from build123d import *

# Parameters (mm, degrees)
F0_R     = 60
F1_DEPTH = 30


with BuildPart() as f1:
    # F0 (on Front) → F1 (new body)
    with BuildSketch(Plane.XZ):
        Polygon((-55, 79.594996), (-125, 79.594996), (-125, 29.594996), (-125, -30.405004), (-125, -80.405004), (-55, -80.405004), (45, -80.405004), (115, -80.405004), (115, -30.405004), (115, 29.594996), (115, 79.594996), (45, 79.594996), align=None)
        with BuildLine():
            ThreePointArc((-110, 55.243649), (-107.071068, 62.314716), (-100, 65.243649))
            Line((-100, 65.243649), (-90, 65.243649))
            ThreePointArc((-90, 65.243649), (-82.928932, 62.314716), (-80, 55.243649))
            Line((-80, 55.243649), (-80, -54.756351))
            ThreePointArc((-80, -54.756351), (-82.928932, -61.827419), (-90, -64.756351))
            Line((-90, -64.756351), (-100, -64.756351))
            ThreePointArc((-100, -64.756351), (-107.071068, -61.827419), (-110, -54.756351))
            Line((-110, -54.756351), (-110, 55.243649))
        make_face(mode=Mode.SUBTRACT)
        Circle(F0_R, mode=Mode.SUBTRACT)
        with BuildLine():
            ThreePointArc((80, 55.243649), (82.928932, 62.314716), (90, 65.243649))
            Line((90, 65.243649), (100, 65.243649))
            ThreePointArc((100, 65.243649), (107.071068, 62.314716), (110, 55.243649))
            Line((110, 55.243649), (110, -54.756351))
            ThreePointArc((110, -54.756351), (107.071068, -61.827419), (100, -64.756351))
            Line((100, -64.756351), (90, -64.756351))
            ThreePointArc((90, -64.756351), (82.928932, -61.827419), (80, -54.756351))
            Line((80, -54.756351), (80, 55.243649))
        make_face(mode=Mode.SUBTRACT)
        with BuildLine():
            Line((-125, -30.405004), (-125, 29.594996))
            ThreePointArc((-125, 29.594996), (-148.860331, -0.405004), (-125, -30.405004))
        make_face()
        with BuildLine():
            ThreePointArc((45, 79.594996), (-5, 105.335071), (-55, 79.594996))
            Line((-55, 79.594996), (45, 79.594996))
        make_face()
        with BuildLine():
            Line((45, -80.405004), (-55, -80.405004))
            ThreePointArc((-55, -80.405004), (-5, -106.628586), (45, -80.405004))
        make_face()
        with BuildLine():
            ThreePointArc((115, -30.405004), (136.54259, -0.405004), (115, 29.594996))
            Line((115, 29.594996), (115, -30.405004))
        make_face()
    extrude(amount=F1_DEPTH)


solid = f1.part
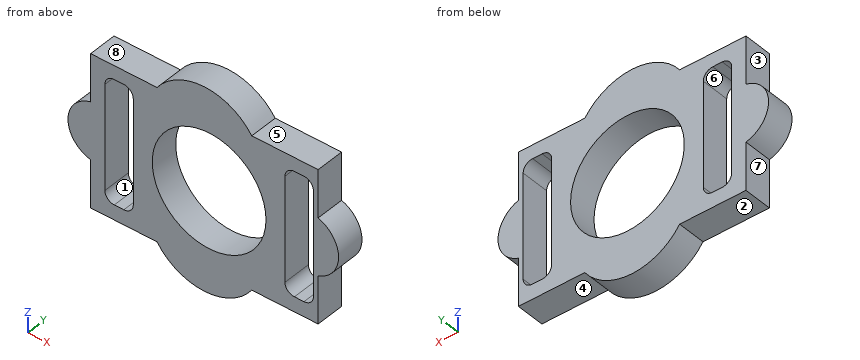
Check sheet for the modelled part. Datum: model origin and axes. Units: mm. Face numbers are marked on the shaded views. A direction names the side the tool comes from. Coordinates: 2 decimals unless noted, no trailing zeros. Write each loop counter-clockwise with the first axis right and the second up, starting at its lowest first coordinate (ties: lowest second). Pieces come first, ordered by that corner, then holes. Notation, with made-up numbers: M 64,14 L 120,14 A23 cw 120,24 Z; hole C 28.5,20 d1. An arc over 180 degrees is marked long. Answer as CSV lines item,"result".
Q1. Mould release check, pull along X, two halves, no side actions. Record for the marked faces 6, 7 and 8: released by +X, released by -X, zero draft, split by the parting line, or undercut.
Check result:
face 6,"undercut"
face 7,"released by -X"
face 8,"zero draft"
Q2. Go/stop test with flat-tipped pins: pin 1 (4 mm diameter, centred on x = -94.5, y = -12.5, fed in from -Z) (3 decimals); pin 2 (6 mm diameter, centred on y = -18, z = 59.5, fed in from +X); pin 3 (15 mm diameter, centred on y = -18, z = -48, fed in from -X). Record where each tip stops, or that it passes through.
Check result:
pin 1,"z = -80.405"
pin 2,"x = 115"
pin 3,"x = -125"
Q3. Cross-section at A-A (y = -26). Count the separate pieces of the cut face and the enclosed holes in it, then the cut area to 3 significant figures.
Check result:
separate pieces,"1"
enclosed holes,"3"
area,"25,100 mm^2"
Q4. Cross-section at C-C (x = -26.5). Record the boundary of the cut face in (y, z), then the cut area to 3 significant figures.
Check result:
outline,"M -30,-102.7 L 0,-102.7 L 0,-53.83 L -30,-53.83 Z; M -30,53.83 L 0,53.83 L 0,101.45 L -30,101.45 Z"
area,"2,890 mm^2"
Q5. Cross-section at B-B (z = -18). Record the boundary of the cut face in (x, y).
Check result:
outline,"M -143.34,-30 L -110,-30 L -110,0 L -143.34,0 Z; M -80,-30 L -57.24,-30 L -57.24,0 L -80,0 Z; M 57.24,-30 L 80,-30 L 80,0 L 57.24,0 Z; M 110,-30 L 131.2,-30 L 131.2,0 L 110,0 Z"
Q6. Cross-section at D-D (z = 37). Record the boundary of the cut face in (x, y).
Check result:
outline,"M -125,-30 L -110,-30 L -110,0 L -125,0 Z; M -80,-30 L -47.23,-30 L -47.23,0 L -80,0 Z; M 47.23,-30 L 80,-30 L 80,0 L 47.23,0 Z; M 110,-30 L 115,-30 L 115,0 L 110,0 Z"
Q7. Material ranges on probe 1 along X at (y, z) = (-9.5, 18); probe 2 along X at (y, z) = (-10.5, 25.5); probe 3 along Z at (x, y) = (94.5, -10) (3 decimals), recorded low to high. Write a range as from..to.
Check result:
probe 1,"-142.75..-110, -80..-57.24, 57.24..80, 110..130.64"
probe 2,"-134.71..-110, -80..-54.31, 54.31..80, 110..123.08"
probe 3,"-80.405..-64.756, 65.244..79.595"
Q8. Set-up check for the marked faces 1, 2, 3, 4 and 5: record each of +Z, -Z, +X, -X, +Y, -Y from which the full face is reachable in a straight line by a thin tool's end or side.
Check result:
face 1,"+Y, -Y"
face 2,"-Z, -X, +Y, -Y"
face 3,"+Z, -X, +Y, -Y"
face 4,"-Z, +X, +Y, -Y"
face 5,"+Z, +X, +Y, -Y"
